from build123d import *

# Parameters (mm, degrees)
F0_W     = 101.6
F0_H     = 165.1
F1_DEPTH = 38.1
F2_W     = 76.2
F2_H     = 139.7
F3_DEPTH = 29.21
F5_DEPTH = 165.1
F8_DEPTH = 177.8
F9_DEPTH = 203.2
F10_R    = 1.905
F11_R    = 1.905


with BuildPart() as f1:
    # F0 (on Top) → F1 (new body)
    with BuildSketch(Plane.XY):
        with Locations((3.219465, 25.661658)):
            Rectangle(F0_W, F0_H)
    extrude(amount=F1_DEPTH)

    # F2 (on face) → F3 (cut)
    with BuildSketch(Plane.XY.offset(38.1)):
        with Locations((3.219465, 25.661658)):
            Rectangle(F2_W, F2_H)
    extrude(amount=-F3_DEPTH, mode=Mode.SUBTRACT)

    # F4 (on face) → F5 (join)
    with BuildSketch(Plane(origin=(0, 108.211658, 0), x_dir=(-1, 0, 0), z_dir=(0, 1, 0))):
        with BuildLine():
            Line((47.580535, 38.1), (47.580535, 0))
            ThreePointArc((47.580535, 0), (57.787384, 19.05), (47.580535, 38.1))
        make_face()
    extrude(amount=-F5_DEPTH)

    # F7 (on face) → F8 (cut)
    with BuildSketch(Plane.YZ.offset(54.019465)):
        with BuildLine():
            ThreePointArc((108.211658, 38.1), (106.126335, 19.05), (108.211658, 0))
            Line((108.211658, 0), (108.211658, 38.1))
        make_face()
        with BuildLine():
            Line((-56.888342, 38.1), (-56.888342, 0))
            ThreePointArc((-56.888342, 0), (-54.735258, 19.05), (-56.888342, 38.1))
        make_face()
    extrude(amount=-F8_DEPTH, mode=Mode.SUBTRACT)

    # F6 (on face) → F9 (cut)
    with BuildSketch(Plane.XZ.offset(56.888342)):
        with BuildLine():
            Line((54.019465, 0), (54.019465, 38.1))
            ThreePointArc((54.019465, 38.1), (52.204457, 19.05), (54.019465, 0))
        make_face()
    extrude(amount=-F9_DEPTH, mode=Mode.SUBTRACT)

    # F10
    f10_edges = [f1.edges().sort_by_distance(p)[0] for p in [
        (52.204457, -54.735258, 19.05),
        (52.204457, 106.126335, 19.05),
    ]]
    fillet(f10_edges, radius=F10_R)

    # F11
    f11_edges = [f1.edges().sort_by_distance(p)[0] for p in [
        (-57.787384, -54.735258, 19.05),
        (-57.787384, 106.126335, 19.05),
    ]]
    fillet(f11_edges, radius=F11_R)


solid = f1.part
Here's how the part is built. I have some questions about the finished solid (model axes, mm). A direction names the side the tool comes from. Round coordinates to 2 decimals unless told otherwise and drop trailing zeros. Order: outer loops, then holes, each group sorted by start corner. A loop starts at its lowest first (then second) coordinate and runs counter-clockwise, first axis right, second up. Notation, with made-up numbers: M 30.5,-1.5 L 57.5,-1.5 A22 cw 57.5,9.5 Z; hole C 13.25,-35 d3. An arc over 180 degrees is marked long. Return JSON: item names as keys, results as strings. Group by question number.
1. If we section it at B-B on y = 53: List the corners of the cut face in (x, z) for me, then the cut area to 3 significant figures.
2. I'm going to push flat-ended pins straight in: pin 1 Ø2 at (y, z) = (43, 16) entering from -X; pin 2 Ø14.5 at (x, z) = (15, 22.5) entering from +Y; pin 3 Ø3 at (y, z) = (-18, 5.5) entering from -X. Where does each tip first touch, or does it pass through?
3. On a 3-axis mill with a long thin cutter (end or side, diameter ignored), from which of +Z, -Z, +X, -X, +Y, -Y can I reach the whole of each face in a straight line? I mean faces 1 (the face through (3, -44.188, 24)), 2 (the face through (-1.104, -54.736, 18.781)). Say none if no direction works.
4. Please list where these lines run through material, in increasing order: probe 1 along X at (y, z) = (-40, 18); probe 2 along Y at (x, z) = (1, 25.5); probe 3 along Y at (x, z) = (16.5, 20).
5. If we section it at C-C on x = -39.5: List the corners of the cut face in (y, z) for me.
6. If we section it at A-A on x = 31.5: List the corners of the cut face in (y, z) for me.
7. If we mould it in two halves opening along X, with no side actions, what happens to faces 3 (the face through (-57.785, 26.792, 18.735)), 4 (the face through (52.205, 24.532, 19.318)), 5 (the face through (3, 95.512, 24)), 6 (the face through (48, 27, 38.1))? For each: pulls with the +X half, pulls with the -X half, needs draft (parallel to the pull), parting line crosses it, or undercut.
Reply:
{
 "1": {"outline": "M -47.58,0 L 54.02,0 A100.88 cw 54.02,38.1 L 41.32,38.1 L 41.32,8.89 L -34.88,8.89 L -34.88,38.1 L -47.58,38.1 A22.88 ccw Z", "area": "1,870 mm^2"},
 "2": {"pin 1": "x = -57.7", "pin 2": "y = 106.78", "pin 3": "x = -54.36"},
 "3": {"face 1": "+Z", "face 2": "+X, -X, -Y"},
 "4": {"probe 1": "-57.76 to -34.88, 41.32 to 52.21", "probe 2": "-54.98 to -44.19, 95.51 to 106.36", "probe 3": "-54.74 to -44.19, 95.51 to 106.13"},
 "5": {"outline": "M -56.89,0 L 108.21,0 A88.06 cw 108.21,38.1 L -56.89,38.1 A85.35 cw Z"},
 "6": {"outline": "M -56.89,0 L 108.21,0 A88.06 cw 108.21,38.1 L 95.51,38.1 L 95.51,8.89 L -44.19,8.89 L -44.19,38.1 L -56.89,38.1 A85.35 cw Z"},
 "7": {"face 3": "pulls with the -X half", "face 4": "pulls with the +X half", "face 5": "undercut", "face 6": "needs draft"}
}
